Build history of the part. All positions in model axes, mm. A direction names the side the tool comes from. Coordinates: 2 decimals unless noted, no trailing zeros. Write each loop counter-clockwise with the first axis right and the second up, starting at its lowest first coordinate (ties: lowest second). Pieces come first, ordered by that corner, then holes.
```python
from build123d import *

# Parameters (mm, degrees)
SKETCH1_R           = 56.769
SKETCH1_R_2         = 52.80025
BOSS_EXTRUDE1_DEPTH = 3.175
SKETCH1_3_R         = 52.80025
BOSS_EXTRUDE2_DEPTH = 3.175
SKETCH2_R           = 12.7
CUT_EXTRUDE1_DEPTH  = 81.534223918


with BuildPart() as part:
    # Sketch1 → Boss-Extrude1 (new body)
    # profile 1 of 2: a face of its own
    with BuildSketch(Plane(origin=(0, 0, 0), x_dir=(1, 0, 0), z_dir=(0, 1, 0))):
        with Locations(Location((0, 0, 0), (0, 0, 270))):
            Circle(SKETCH1_R)
        Circle(SKETCH1_R_2, mode=Mode.SUBTRACT)
    # profile 2 of 2: a face of its own
    with BuildSketch(Plane(origin=(0, 0, 0), x_dir=(1, 0, 0), z_dir=(0, 1, 0))):
        Circle(SKETCH1_R_2)
    extrude(amount=BOSS_EXTRUDE1_DEPTH)

    # Sketch1_3 → Boss-Extrude2 (add)
    with BuildSketch(Plane(origin=(0, 0, 0), x_dir=(1, 0, 0), z_dir=(0, 1, 0))):
        with Locations(Location((0, 0, 0), (0, 0, 270))):
            Circle(SKETCH1_3_R)
    extrude(amount=-BOSS_EXTRUDE2_DEPTH)

    # Sketch2 → Cut-Extrude1 (cut, through all)
    with BuildSketch(Plane(origin=(0, 3.175, 0), x_dir=(1, 0, 0), z_dir=(0, 1, 0))):
        with Locations(Location((0, 31.75, 0), (0, 0, 270))):
            Circle(SKETCH2_R)
        with Locations(Location((28.575, 3.175, 0), (0, 0, 270))):
            Circle(SKETCH2_R)
        with Locations(Location((0, -25.4, 0), (0, 0, 270))):
            Circle(SKETCH2_R)
        with Locations(Location((-28.575, 3.175, 0), (0, 0, 270))):
            Circle(SKETCH2_R)
    extrude(amount=-CUT_EXTRUDE1_DEPTH, mode=Mode.SUBTRACT)


solid = part.part
```
1. Probe line 1 along Z through (x, y) = (4.5, 0.5); line 2 along X through (y, z) = (-1, 30); line 3 along X through (y, z) = (-0.5, -35.5). List the from-to ranges inside material, lowest first.
Computed values:
line 1: z = -56.59 to -43.63, -19.87 to 13.52, 37.28 to 56.59
line 2: x = -43.45 to -11.84, 11.84 to 43.45
line 3: x = -39.08 to -12.13, 12.13 to 39.08
2. Flat gauge pins, fed straight in: pin 1 (2 mm diameter, centred on x = -17, y = 1, fed in from -Z); pin 2 (10 mm diameter, centred on x = 44.5, z = -36.5, fed in from +Y) (3 decimals); pin 3 (1.5 mm diameter, centred on y = -0.5, z = 21, fed in from -X). Where does each tip first touch, or does it go through?
Computed values:
pin 1: stops at z = -54.47
pin 2: stops at y = 3.175
pin 3: stops at x = -52.96
3. 3-axis set-ups, long thin cutter, end or side, ignore diameter. For faces 1 (the face through (38, 0, 38)), 2 (the face through (1, -3.175, -1)): which of +Z, -Z, +X, -X, +Y, -Y reach the whole face in a straight line?
Computed values:
face 1: -Y
face 2: +Z, -Z, +X, -X, -Y
4. Saw through at B-B on z = 0. List the corners of the cut face in (x, y) (3 decimals), plus the area to 3 significant figures.
Computed values:
outline: (-56.769, 0) - (-52.8, 0) - (-52.8, -3.175) - (-40.872, -3.175) - (-40.872, 3.175) - (-56.769, 3.175) - close; (-16.278, -3.175) - (16.278, -3.175) - (16.278, 3.175) - (-16.278, 3.175) - close; (40.872, -3.175) - (52.8, -3.175) - (52.8, 0) - (56.769, 0) - (56.769, 3.175) - (40.872, 3.175) - close
area: 383 mm2
5. Saw through at A-A on x = 0. List the corners of the cut face in (y, z) (3 decimals).
Computed values:
outline: (-3.175, -52.8) - (0, -52.8) - (0, -56.769) - (3.175, -56.769) - (3.175, -44.45) - (-3.175, -44.45) - close; (-3.175, -19.05) - (3.175, -19.05) - (3.175, 12.7) - (-3.175, 12.7) - close; (-3.175, 38.1) - (3.175, 38.1) - (3.175, 56.769) - (0, 56.769) - (0, 52.8) - (-3.175, 52.8) - close
6. Saw through at C-C on z = -31.75. List the corners of the cut face in (x, y) (3 decimals), plus the area to 3 significant figures.
Computed values:
outline: (-47.06, 0) - (-42.188, 0) - (-42.188, -3.175) - (-12.7, -3.175) - (-12.7, 3.175) - (-47.06, 3.175) - close; (12.7, -3.175) - (42.188, -3.175) - (42.188, 0) - (47.06, 0) - (47.06, 3.175) - (12.7, 3.175) - close
area: 405 mm2
7. Mould opens along X. For faces 3 (the face through (-32, -2, -42)), 4 (the face through (0.558, 0.044, 12.712)), 5 (the face through (1, 3.175, -1)) say: +X half, -X half, draft (parallel to the pull), parting line (faces both ways), or undercut.
Computed values:
face 3: parting line
face 4: undercut
face 5: draft
8. Saw through at D-D on x = -19. List the corners of the cut face in (y, z) (3 decimals).
Computed values:
outline: (-3.175, -49.263) - (0, -49.263) - (0, -53.495) - (3.175, -53.495) - (3.175, -11.518) - (-3.175, -11.518) - close; (-3.175, 5.168) - (3.175, 5.168) - (3.175, 53.495) - (0, 53.495) - (0, 49.263) - (-3.175, 49.263) - close
